Geometry: final body of the model. Coordinates: model frame, mm. A direction names the side the tool comes from. Give positions to 0.01 mm unless a question says otherwise; leave off trailing zeros. Write each loop counter-clockwise with the first axis right and the second up, starting at its lowest first coordinate (ties: lowest second). Pieces come first, ordered by that corner, then holes. Notation, with made-up numbers: (-21.75, -15.5) -> (-17.75, -15.5) arc R24 ccw to (-17.75, 21.5) -> close; hole circle Ø4 at (-13, 77). An arc over 180 degrees is marked (long way). Answer in a Markdown table with one row per item. Add a question column.
Item 1: Draft query along X for faces 4 (the cylindrical face through (-155.44, 177.27, -1704.43)), 5 (the cylindrical face through (-209.887, 177.876, -1333.848)), 6 (the flat face through (-230, 139.7, -1658)), 7 (the cylindrical face through (-277.158, 177.267, -1664.999)). Return one class per face: +X half, -X half, draft (parallel to the pull), parting line (faces both ways), or undercut.
Item 2: Section query B-B on z = -1272.5. Output: boundary loops of the cut face in (x, y), plus the area to 3 significant figures.
Item 3: Section query D-D on y = 148.5. Output: boundary loops of the cut face in (x, z), plus the area to 3 significant figures.
Item 4: Section query A-A on x = -157.5. Output: boundary loops of the cut face in (y, z).
Item 5: Material intervals for probe 1 along Z at (x, y) = (-176, 180); probe 2 along X at (y, z) = (186.5, -1848); probe 3 along X at (y, z) = (154, -1592), sorted ascending. Write a range as from..to.
Item 6: Section query C-C on x = -200.5. Output: boundary loops of the cut face in (y, z), plus the area to 3 significant figures.
Item 7: First-contact query: P1, Ø4, axis at y = 204.5, z = -1856.5, coming from the +X side; P2, Ø3, axis at x = -343, y = 207.5, coming from the -Z side; P3, Ø10, axis at y = 202.5, z = -1735, coming from the -X side. Flat tips, straight axial feed; report the tip coordinate or a pass-through.
Item 8: Access query for faces 1 (the flat face through (-230, 215.9, -1658)), 2 (the flat face through (-229, 183.243, -1309)), 3 (the flat face through (-229, 172.357, -1273)). Directions: +Z, -Z, +X, -X, +Y, -Y. A direction counts if a zero-diameter tool reaches every point of the face in a straight line with its end or side. Return the directions, or none.
```python
from build123d import *

# Parameters (mm, degrees)
BOSS_EXTRUDE1_DEPTH = 355.6
CUT_EXTRUDE2_START  = -152.4
SKETCH5_R           = 355.6
CUT_EXTRUDE2_DEPTH  = 152.4
SKETCH6_R           = 355.6
CUT_EXTRUDE3_DEPTH  = 152.4
SKETCH7_R           = 254
CUT_EXTRUDE4_DEPTH  = 152.4
CUT_EXTRUDE5_DEPTH  = 635
SCALE1_SCALE        = 0.214285714


with BuildPart() as part:
    # Sketch2 → Boss-Extrude1 (new body)
    with BuildSketch(Plane(origin=(0, 0, 0), x_dir=(1, 0, 0), z_dir=(0, 1, 0))):
        with BuildLine():
            ThreePointArc((-285.969579472, 211.359314005), (160.143666656, -317.498607918), (0, 355.6))
            ThreePointArc((0, 355.6), (92.407240491, 1952.73574683), (-939.8, 3175))
            ThreePointArc((-939.8, 3175), (-1137.137455821, 1577.520446779), (-285.969579472, 211.359314005))
        make_face()
    extrude(amount=BOSS_EXTRUDE1_DEPTH)

    # Sketch5 → Cut-Extrude2 (cut)
    with BuildSketch(Plane(origin=(0, 355.6, 0), x_dir=(1, 0, 0), z_dir=(0, 1, 0)).offset(CUT_EXTRUDE2_START)):
        Circle(SKETCH5_R)
    extrude(amount=CUT_EXTRUDE2_DEPTH, mode=Mode.SUBTRACT)

    # Sketch6 → Cut-Extrude3 (cut)
    with BuildSketch(Plane.XZ):
        Circle(SKETCH6_R)
    extrude(amount=-CUT_EXTRUDE3_DEPTH, mode=Mode.SUBTRACT)

    # Sketch7 → Cut-Extrude4 (cut)
    with BuildSketch(Plane(origin=(0, 203.2, 0), x_dir=(1, 0, 0), z_dir=(0, 1, 0))):
        with Locations(Location((0, 0, 0), (0, 0, 270))):
            Circle(SKETCH7_R)
    extrude(amount=-CUT_EXTRUDE4_DEPTH, mode=Mode.SUBTRACT)

    # Sketch8 → Cut-Extrude5 (cut)
    with BuildSketch(Plane.XZ):
        with BuildLine():
            ThreePointArc((-939.8, -3175), (-463.84673696, -1726.060030518), (-285.969579472, -211.359314005))
            ThreePointArc((-285.969579472, -211.359314005), (-1137.137455821, -1577.520446779), (-939.8, -3175))
        make_face()
    extrude(amount=-CUT_EXTRUDE5_DEPTH, mode=Mode.SUBTRACT)


with BuildPart() as part_1:
    # Scale1: scaled about (-224.977664094, 177.8, -1642.651878674)
    add(part.part.scale(SCALE1_SCALE).moved(Location((-176.768164645, 139.7, -1290.65504753))))


solid = part_1.part
```
Findings below:
| question | item | result |
|---|---|---|
| 1 | face 4 | +X half |
| 1 | face 5 | undercut |
| 1 | face 6 | draft |
| 1 | face 7 | -X half |
| 2 | outline | (-250.77, 172.36) -> (-228.08, 172.36) -> (-228.08, 183.24) -> (-250.77, 183.24) -> close; (-125.46, 172.36) -> (-102.76, 172.36) -> (-102.76, 183.24) -> (-125.46, 183.24) -> close |
| 2 | area | 494 mm^2 |
| 3 | outline | (-378.15, -1971.01) arc R462.64 ccw to (-176.77, -1366.86) arc R76.2 cw to (-238.05, -1335.95) arc R1632.86 cw to start |
| 3 | area | 62,600 mm^2 |
| 4 | outline | (139.7, -1710.69) -> (215.9, -1710.69) -> (215.9, -1414.91) -> (139.7, -1414.91) -> close; (172.36, -1364.38) -> (183.24, -1364.38) -> (183.24, -1341.56) -> (172.36, -1341.56) -> close; (172.36, -1239.75) -> (183.24, -1239.75) -> (183.24, -1216.93) -> (172.36, -1216.93) -> close |
| 5 | probe 1 | z = -1757.09..-1368.51, -1366.85..-1345.08, -1236.23..-1214.46 |
| 5 | probe 2 | x = -329.44..-231.59 |
| 5 | probe 3 | x = -262.58..-134.15 |
| 6 | outline | (139.7, -1803.05) -> (215.9, -1803.05) -> (215.9, -1363.07) -> (183.24, -1363.07) -> (183.24, -1339.64) -> (172.36, -1339.64) -> (172.36, -1363.07) -> (139.7, -1363.07) -> close; (172.36, -1241.67) -> (183.24, -1241.67) -> (183.24, -1218.24) -> (172.36, -1218.24) -> close |
| 6 | area | 34,000 mm^2 |
| 7 | P1 | stops at x = -236.77 |
| 7 | P2 | stops at z = -1951.2 |
| 7 | P3 | stops at x = -295.8 |
| 8 | face 1 | +Z, -Z, +X, -X, +Y |
| 8 | face 2 | +Z, +X, +Y |
| 8 | face 3 | +Z, +X, -Y |
